Source: three-view drawing plus pictorial views. Frame: mm from the lowest corner of the part. Give positions to 0.01 mm unless a question says otherwise; leave off trailing zeros. Loops run counter-clockwise (first coordinate to the right, second up) from the corner with the lowest first, then second, coordinate; pieces in that order, holes last. Notation, with made-up numbers: (-15.5, 66) - (-2.5, 66) arc R18 cw to (-2.5, 92) - close; hole circle Ø3 at (26.5, 49.25). An arc over 180 degrees is marked (long way). Put each result on its own line as item: value.
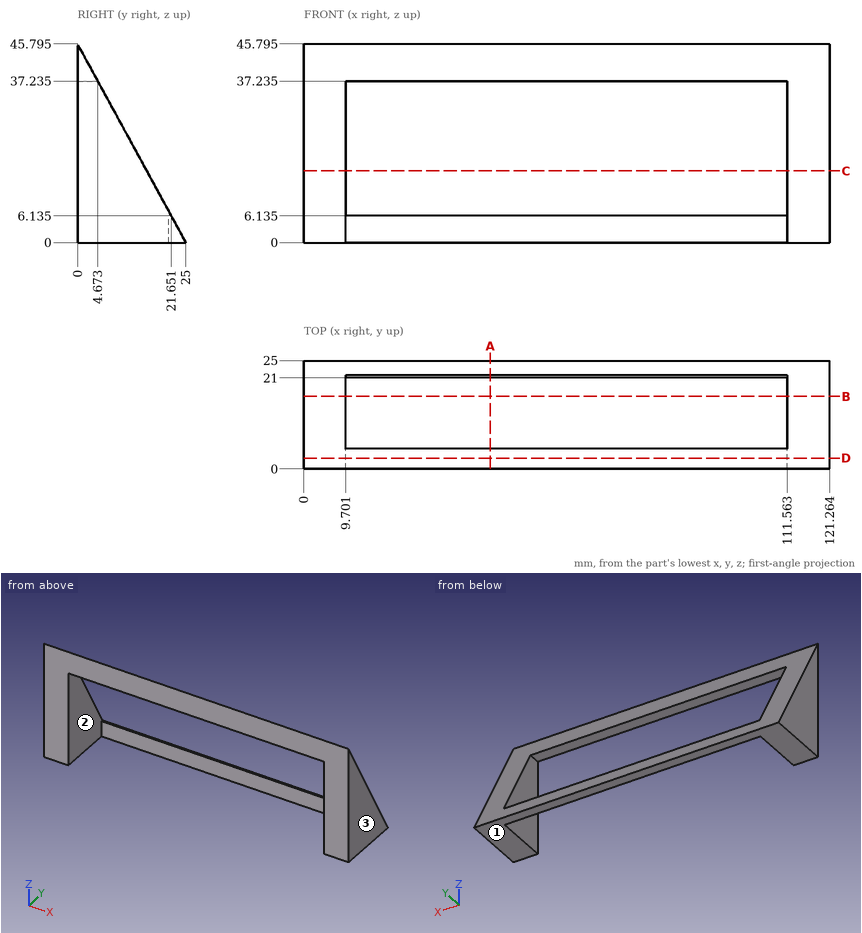
1) Mould query, pull axis X, two halves, no side actions, for the marked faces 1, 2 and 3. Classes: pulls with the +X half, pulls with the -X half, needs draft (parallel to the pull), parting line crosses it, or undercut.
Check result:
face 1: needs draft
face 2: undercut
face 3: pulls with the +X half
2) Section query B-B, the plane y = 16.75. Output: boundary loops of the cut face in (x, z), plus the area to 3 significant figures.
Check result:
outline: (0, 0) - (9.7, 0) - (9.7, 15.11) - (0, 15.11) - close; (111.56, 0) - (121.26, 0) - (121.26, 15.11) - (111.56, 15.11) - close
area: 293 mm²
3) Section query A-A, the plane x = 43. Output: boundary loops of the cut face in (y, z) (1 decimal).
Check result:
outline: (0, 37.2) - (4.7, 37.2) - (0, 45.8) - close; (21, 0) - (25, 0) - (21.7, 6.1) - (21, 6.1) - close
4) Section query D-D, the plane y = 2.5. Output: boundary loops of the cut face in (x, z) (1 decimal).
Check result:
outline: (0, 0) - (9.7, 0) - (9.7, 37.2) - (111.6, 37.2) - (111.6, 0) - (121.3, 0) - (121.3, 41.2) - (0, 41.2) - close
5) Material intervals for line 1 along X through (y, z) = (10.75, 22); line 2 along Z through (x, y) = (82.5, 21.5) (1 decimal); line 3 along Z through (x, y) = (30, 2.5) (1 decimal), sorted ascending. Write a range as [from, to].
Check result:
line 1: [0, 9.7], [111.56, 121.26]
line 2: [0, 6.1]
line 3: [37.2, 41.2]
6) Pin query (flat end, axial travel): P1, Ø6, axis at x = 24, y = 6, coming from the -Z side (1 decimal); P2, Ø0.5, axis at x = 74.5, y = 21.5, coming from the +Z side (1 decimal); P3, Ø5, axis at x = 43, z = 4.5, coming from the -Y side. Return the tip coordinate at first contact, or that it passes through.
Check result:
P1: z = 37.2
P2: z = 6.1
P3: y = 21
7) Section query C-C, the plane z = 16.5. Output: boundary loops of the cut face in (x, y).
Check result:
outline: (0, 0) - (9.7, 0) - (9.7, 15.99) - (0, 15.99) - close; (111.56, 0) - (121.26, 0) - (121.26, 15.99) - (111.56, 15.99) - close
